Input: dimensioned drawing with shaded views. Units: mm. Origin: part minimum x, y, z. A direction names the side the tool comes from. Coordinates: 2 decimals unless noted, no trailing zeros. Loops run counter-clockwise (first coordinate to the right, second up) from the corner with the lowest first, then second, coordinate; pieces in that order, holes last. Notation, with made-up numbers: (38.5, -38) - (54.5, -38) arc R21 cw to (54.5, -25) - close; hole circle Ø5 at (66.25, -19). An arc over 180 degrees is marked (long way). Put each result on its own line as item: value. Start each with the question number.
1) Section A-A on z = 35. Output: boundary loops of the cut face in (x, y) (1 decimal), and give its area (3 significant figures).
2) Section C-C on x = 1349.5. Output: boundary loops of the cut face in (y, z).
3) Section B-B on y = 540. Output: boundary loops of the cut face in (x, z) (1 decimal), and give its area (3 significant figures).
4) Section D-D on x = 1173. Output: boundary loops of the cut face in (y, z).
5) Reachability of the marked faces 5, 6 and 7 from +Z, -Z, +X, -X, +Y, -Y: full face, straight path, thin tool, end or side. Return the list, or none.
6) Draft query along X for the marked faces 1, 2, 3 and 4. Return one class per face: +X half, -X half, draft (parallel to the pull), parting line (faces both ways), or undercut.
7) Contact query for flat-ended pins moving along their axis: pin 1 Ø8 at (x, y) = (361.5, 259.5) entering from +Z; pin 2 Ø1.5 at (x, z) = (626.5, 34) entering from -Y. Output: stop coordinate, or through.
8) Material intervals for line 1 along X through (y, z) = (471, 30) (1 decimal); line 2 along Z through (x, y) = (1525, 329.5); line 3 along Y through (x, z) = (76, 22), sorted ascending. Write a range as from..to.
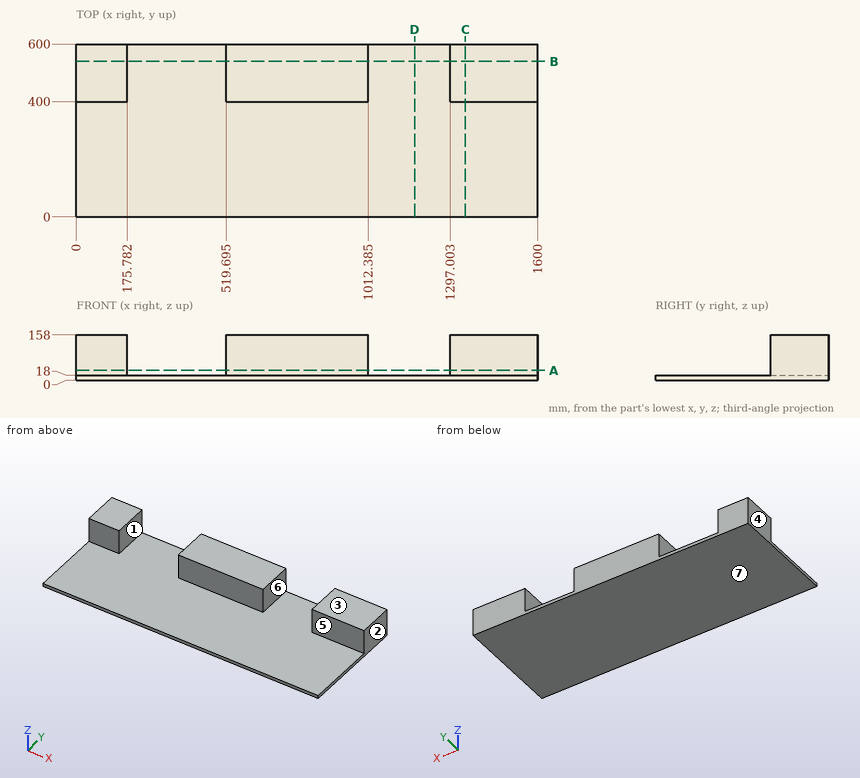
Answer block:
1. outline: (0, 400) - (175.8, 400) - (175.8, 600) - (0, 600) - close; (519.7, 400) - (1012.4, 400) - (1012.4, 600) - (519.7, 600) - close; (1297, 400) - (1600, 400) - (1600, 600) - (1297, 600) - close
1. area: 194,000 mm²
2. outline: (0, 0) - (600, 0) - (600, 158) - (400, 158) - (400, 18) - (0, 18) - close
3. outline: (0, 0) - (1600, 0) - (1600, 158) - (1297, 158) - (1297, 18) - (1012.4, 18) - (1012.4, 158) - (519.7, 158) - (519.7, 18) - (175.8, 18) - (175.8, 158) - (0, 158) - close
3. area: 165,000 mm²
4. outline: (0, 0) - (600, 0) - (600, 18) - (0, 18) - close
5. face 5: +Z, +X, -X, -Y
5. face 6: +Z, +Y, -Y
5. face 7: -Z, +X, -X, +Y, -Y
6. face 1: undercut
6. face 2: +X half
6. face 3: draft
6. face 4: -X half
7. pin 1: stops at z = 18
7. pin 2: stops at y = 400
8. line 1: x = 0..175.8, 519.7..1012.4, 1297..1600
8. line 2: z = 0..18
8. line 3: y = 400..600
